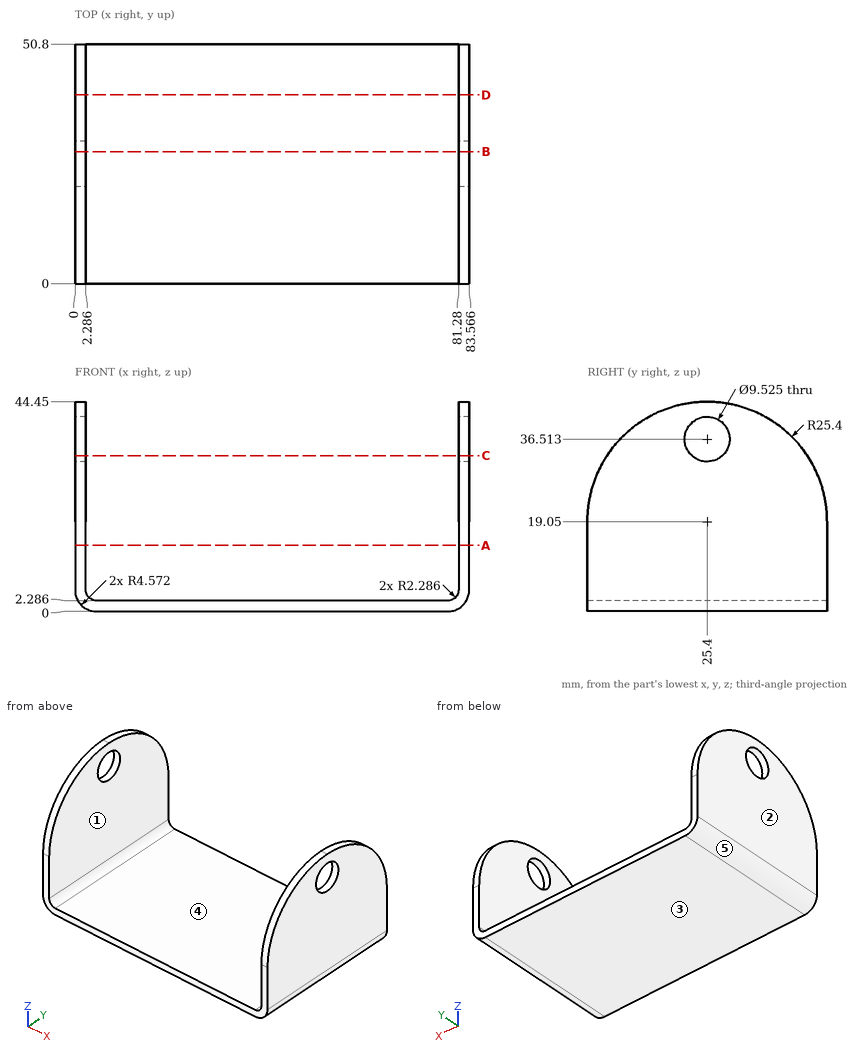
Drawing for the job (mm, zero at the part's lowest x, y, z). A direction names the side the tool comes from. Give positions to 0.01 mm unless a question says otherwise; leave off trailing zeros. Loops run counter-clockwise (first coordinate to the right, second up) from the corner with the lowest first, then second, coordinate; pieces in that order, holes last.
Item 1: Slice it at A-A (z = 14). Write the cut outline in (x, y) (1 decimal), plus the area to 3 significant figures.
Check values:
outline: (0, 0) - (2.3, 0) - (2.3, 50.8) - (0, 50.8) - close; (81.3, 0) - (83.6, 0) - (83.6, 50.8) - (81.3, 50.8) - close
area: 232 mm2
Item 2: Slice it at C-C (z = 33). Write the cut outline in (x, y) (1 decimal), plus the area to 3 significant figures.
Check values:
outline: (0, 4.2) - (2.3, 4.2) - (2.3, 22.2) - (0, 22.2) - close; (0, 28.6) - (2.3, 28.6) - (2.3, 46.6) - (0, 46.6) - close; (81.3, 4.2) - (83.6, 4.2) - (83.6, 22.2) - (81.3, 22.2) - close; (81.3, 28.6) - (83.6, 28.6) - (83.6, 46.6) - (81.3, 46.6) - close
area: 165 mm2
Item 3: Slice it at D-D (y = 40). Write the cut outline in (x, z) (1 decimal).
Check values:
outline: (0, 4.6) arc R4.6 ccw to (4.6, 0) - (79, 0) arc R4.6 ccw to (83.6, 4.6) - (83.6, 39.8) - (81.3, 39.8) - (81.3, 4.6) arc R2.3 cw to (79, 2.3) - (4.6, 2.3) arc R2.3 cw to (2.3, 4.6) - (2.3, 39.8) - (0, 39.8) - close
Item 4: Drop flat-ended pins along their axis: P1, Ø6, axis at x = 30, y = 8, coming from the +Z side; P2, Ø15, axis at y = 25.4, z = 36.51, coming from the -X side. Give the stop position or say it passes through.
Check values:
P1: stops at z = 2.29
P2: stops at x = 0
Item 5: Drill centre lines: line 1 along X through (y, z) = (29, 42.5) (1 decimal); line 2 along Z through (x, y) = (33, 2) (1 decimal); line 3 along X through (y, z) = (19, 4) (1 decimal). Where is each one in solid material? Low to high.
Check values:
line 1: x = 0 to 2.3, 81.3 to 83.6
line 2: z = 0 to 2.3
line 3: x = 0 to 2.4, 81.2 to 83.5
Item 6: Mould opens along X. For the marked faces 3, 4 and 5 say: +X half, -X half, draft (parallel to the pull), parting line (faces both ways), or undercut.
Check values:
face 3: draft
face 4: undercut
face 5: -X half
Item 7: Which spindle directions (+Z, -Z, +X, -X, +Y, -Y) get a long thin tool onto all of the face, cutting with end or side? Do the marked faces 1 and 2. Say none if no direction does.
Check values:
face 1: +Z, +Y, -Y
face 2: +Z, -Z, -X, +Y, -Y
Item 8: Slice it at B-B (y = 28). Write the cut outline in (x, z) (1 decimal).
Check values:
outline: (0, 4.6) arc R4.6 ccw to (4.6, 0) - (79, 0) arc R4.6 ccw to (83.6, 4.6) - (83.6, 32.5) - (81.3, 32.5) - (81.3, 4.6) arc R2.3 cw to (79, 2.3) - (4.6, 2.3) arc R2.3 cw to (2.3, 4.6) - (2.3, 32.5) - (0, 32.5) - close; (0, 40.5) - (2.3, 40.5) - (2.3, 44.3) - (0, 44.3) - close; (81.3, 40.5) - (83.6, 40.5) - (83.6, 44.3) - (81.3, 44.3) - close
